CAD build for the part. Positions are in the model's coordinates, mm. A direction names the side the tool comes from. Give positions to 0.01 mm unless a question says otherwise; leave off trailing zeros. Loops run counter-clockwise (first coordinate to the right, second up) from the corner with the lowest first, then second, coordinate; pieces in that order, holes last. Notation, with made-up numbers: M 74.25,30 L 98.25,30 A33 cw 98.25,67 Z; hole C 68,39.5 d9. An arc over 180 degrees is marked long. Answer as CSV lines item,"result".
from build123d import *

# Parameters (mm, degrees)
SKETCH1_W                    = 31.75
SKETCH1_H                    = 1.5875
BOSS_EXTRUDE1_DEPTH          = 44.45
SKETCH2_W                    = 31.75
SKETCH2_H                    = 1.5875
BOSS_EXTRUDE2_DEPTH          = 31.75
SKETCH3_R                    = 9.525
CUT_EXTRUDE1_DEPTH           = 64.994170877
F_3_0_3_DIAMETER_HOLE1_D     = 3
F_3_0_3_DIAMETER_HOLE1_DEPTH = 3.556
F_3_0_3_DIAMETER_HOLE1_TIP   = 0.901290929
F_3_0_3_DIAMETER_HOLE2_D     = 3
F_3_0_3_DIAMETER_HOLE2_DEPTH = 3.556
F_3_0_3_DIAMETER_HOLE2_TIP   = 0.901290929


with BuildPart() as part:
    # Sketch1 → Boss-Extrude1 (new body)
    with BuildSketch(Plane.XY):
        with Locations((15.875, 0.79375)):
            Rectangle(SKETCH1_W, SKETCH1_H)
    extrude(amount=BOSS_EXTRUDE1_DEPTH)

    # Sketch2 → Boss-Extrude2 (add)
    with BuildSketch(Plane(origin=(0, 1.5875, 0), x_dir=(1, 0, 0), z_dir=(0, 1, 0))):
        with Locations((15.875, -0.79375)):
            Rectangle(SKETCH2_W, SKETCH2_H)
    extrude(amount=BOSS_EXTRUDE2_DEPTH)

    # Sketch3 → Cut-Extrude1 (cut, through all)
    with BuildSketch(Plane(origin=(0, 0, 0), x_dir=(-1, 0, 0), z_dir=(0, 0, -1))):
        with Locations((-15.875, 17.78)):
            Circle(SKETCH3_R)
    extrude(amount=-CUT_EXTRUDE1_DEPTH, mode=Mode.SUBTRACT)

    # Ø3.0 (3) Diameter Hole1
    with Locations(Plane(origin=(0, 0, 0), x_dir=(-1, 0, 0), z_dir=(0, 0, -1))):
        with Locations((-15.875, 30.226), (-15.875, 5.334)):
            Hole(F_3_0_3_DIAMETER_HOLE1_D / 2, depth=F_3_0_3_DIAMETER_HOLE1_DEPTH)
            with Locations((0, 0, -(F_3_0_3_DIAMETER_HOLE1_DEPTH + F_3_0_3_DIAMETER_HOLE1_TIP / 2))):  # 118° drill point
                Cone(0, F_3_0_3_DIAMETER_HOLE1_D / 2, F_3_0_3_DIAMETER_HOLE1_TIP, mode=Mode.SUBTRACT)

    # Ø3.0 (3) Diameter Hole2
    with Locations(Plane(origin=(0, 1.5875, 0), x_dir=(1, 0, 0), z_dir=(0, 1, 0))):
        with Locations((22.225, -12.7), (22.225, -35.469930371), (9.525, -12.7), (9.525, -35.56)):
            Hole(F_3_0_3_DIAMETER_HOLE2_D / 2, depth=F_3_0_3_DIAMETER_HOLE2_DEPTH)
            with Locations((0, 0, -(F_3_0_3_DIAMETER_HOLE2_DEPTH + F_3_0_3_DIAMETER_HOLE2_TIP / 2))):  # 118° drill point
                Cone(0, F_3_0_3_DIAMETER_HOLE2_D / 2, F_3_0_3_DIAMETER_HOLE2_TIP, mode=Mode.SUBTRACT)


solid = part.part
1) Band-saw the part on B-B on z = 12.7. Give the number of separate pieces and of enclosed holes in the cut face, and give its area (3 significant figures).
Answer below:
separate pieces,"3"
enclosed holes,"0"
area,"40.9 mm^2"
2) Drill centre lines: line 1 (X direction, y = 0.5, z = 35.56) (3 decimals); line 2 (Z direction, x = 19, y = 4.5). Where is each one in solid material? Low to high. Write a range as from..to.
Answer below:
line 1,"x = 0..8.025, 11.025..20.728, 23.722..31.75"
line 2,"z = 0..1.59"
3) Which spindle directions (+Z, -Z, +X, -X, +Y, -Y) get a long thin tool onto all of the face, cutting with end or side? Do faces 4 (the face through (20.839, 0.783, 13.275)), 5 (the face through (9, 10, 1.588)). Say none if no direction does.
Answer below:
face 4,"+Y, -Y"
face 5,"+Z, +X, -X, +Y"
4) Band-saw the part on C-C on x = 23. Give the cut face in (y, z), and give its area (3 significant figures).
Answer below:
outline,"M 0,0 L 11.46,0 L 11.46,1.59 L 1.59,1.59 L 1.59,11.42 L 0,11.42 Z; M 0,13.98 L 1.59,13.98 L 1.59,34.19 L 0,34.19 Z; M 0,36.75 L 1.59,36.75 L 1.59,44.45 L 0,44.45 Z; M 24.1,0 L 33.34,0 L 33.34,1.59 L 24.1,1.59 Z"
area,"92.7 mm^2"
5) Flat gauge pins, fed straight in: pin 1 (3.5 mm diameter, centred on x = 15.875, y = 30.226, fed in from +Z); pin 2 (5 mm diameter, centred on x = 9.525, z = 35.56, fed in from +Y). Where does each tip first touch, or does it go through?
Answer below:
pin 1,"stops at z = 1.59"
pin 2,"stops at y = 1.59"
6) Band-saw the part on A-A on y = 17.78. Give the cut face in (x, z), and give its area (3 significant figures).
Answer below:
outline,"M 0,0 L 6.35,0 L 6.35,1.59 L 0,1.59 Z; M 25.4,0 L 31.75,0 L 31.75,1.59 L 25.4,1.59 Z"
area,"20.2 mm^2"
7) Mould opens along X. For faces 1 (the face through (16, 1.588, 23)), 2 (the face through (0, 1, 12)), 3 (the face through (14.376, 5.4, 0.805)) say: +X half, -X half, draft (parallel to the pull), parting line (faces both ways), or undercut.
Answer below:
face 1,"draft"
face 2,"-X half"
face 3,"undercut"
8) Band-saw the part on D-D on y = 23. Give the cut face in (x, z), and give its area (3 significant figures).
Answer below:
outline,"M 0,0 L 7.91,0 L 7.91,1.59 L 0,1.59 Z; M 23.84,0 L 31.75,0 L 31.75,1.59 L 23.84,1.59 Z"
area,"25.1 mm^2"
